```python
from build123d import *

# Parameters (mm, degrees)
CROQUIS1_W              = 600
CROQUIS1_H              = 250
CROQUIS1_W_2            = 80
CROQUIS1_H_2            = 150
SALIENTE_EXTRUIR2_DEPTH = 25
CORTAR_EXTRUIR2_REACH   = 252
CROQUIS3_R              = 6.5


with BuildPart() as part:
    # Croquis1 → Saliente-Extruir2 (new body)
    with BuildSketch(Plane.XY):
        Rectangle(CROQUIS1_W, CROQUIS1_H)
        with Locations((0, -30)):
            Rectangle(CROQUIS1_W_2, CROQUIS1_H_2, mode=Mode.SUBTRACT)
    extrude(amount=SALIENTE_EXTRUIR2_DEPTH)

    # Croquis3 → Cortar-Extruir2 (cut, up to next)
    with BuildSketch(Plane.XZ.offset(125), mode=Mode.PRIVATE) as cortar_extruir2_sk1:
        with Locations((0, 12.5)):
            Circle(CROQUIS3_R)
    cortar_extruir2_tool1 = extrude(cortar_extruir2_sk1.sketch, amount=-CORTAR_EXTRUIR2_REACH, mode=Mode.PRIVATE) & part.part
    add(cortar_extruir2_tool1.solids().sort_by_distance((0, -125, 12.5))[0], mode=Mode.SUBTRACT)


solid = part.part
```
Verification items for the finished model (mm, model axes). A direction names the side the tool comes from. Coordinates: 2 decimals unless noted, no trailing zeros. Order: outer loops, then holes, each group sorted by start corner. A loop starts at its lowest first (then second) coordinate and runs counter-clockwise, first axis right, second up. Notation, with made-up numbers: (84.5, 71) - (115.5, 71) arc R20 ccw to (115.5, 81) - close; hole circle Ø11 at (60.5, -34). An arc over 180 degrees is marked (long way). Return JSON: item names as keys, results as strings.
(1) Access from +Z, -Z, +X, -X, +Y, -Y to the whole of each face (thin tool, end or side, straight path). Record for faces 4 (the flat face through (-4, -125, 7)), 5 (the flat face through (-1, -105, 4)), 6 (the cylindrical face through (3.494, -115.14, 17.981)).
Filled sheet:
{"face 4": "+Z, -Z, +X, -X, -Y", "face 5": "+Z, -Z", "face 6": "-Y"}
(2) Mould release check, pull along X, two halves, no side actions. Record for faces 1 (the flat face through (-300, -2, 12)), 2 (the flat face through (-40, -31, 12)), 3 (the flat face through (-4, 57, 0)): pulls with the +X half, pulls with the -X half, needs draft (parallel to the pull), parting line crosses it, or undercut.
Filled sheet:
{"face 1": "pulls with the -X half", "face 2": "undercut", "face 3": "needs draft"}
(3) Thickness scan on line 1 along Z through (x, y) = (0, -121); line 2 along X through (y, z) = (-76, 4). Record the ranges inside material, lowest first.
Filled sheet:
{"line 1": "z = 0 to 6, 19 to 25", "line 2": "x = -300 to -40, 40 to 300"}
(4) Section check A-A, the plane x = -25. Record the cut outline in (y, z).
Filled sheet:
{"outline": "(-125, 0) - (-105, 0) - (-105, 25) - (-125, 25) - close; (45, 0) - (125, 0) - (125, 25) - (45, 25) - close"}
(5) Section check B-B, the plane y = 6. Record the cut outline in (x, z).
Filled sheet:
{"outline": "(-300, 0) - (-40, 0) - (-40, 25) - (-300, 25) - close; (40, 0) - (300, 0) - (300, 25) - (40, 25) - close"}
(6) Section check C-C, the plane z = 12.5. Record the cut outline in (x, y), and give its area (3 significant figures).
Filled sheet:
{"outline": "(-300, -125) - (-6.5, -125) - (-6.5, -105) - (-40, -105) - (-40, 45) - (40, 45) - (40, -105) - (6.5, -105) - (6.5, -125) - (300, -125) - (300, 125) - (-300, 125) - close", "area": "138,000 mm^2"}
